Geometry check sheet. Reference: the model listing, model coordinates, mm. A direction names the side the tool comes from. Give positions to 0.01 mm unless a question says otherwise; leave off trailing zeros. Order: outer loops, then holes, each group sorted by start corner. A loop starts at its lowest first (then second) coordinate and runs counter-clockwise, first axis right, second up.
from build123d import *

# Parameters (mm, degrees)
F1_DEPTH = 25
F2_R     = 3
F3_DEPTH = 15


with BuildPart() as f1:
    # F0 (on Top) → F1 (new body)
    with BuildSketch(Plane.XY):
        with BuildLine():
            Line((5.183941, -22.5), (6.75, -22.5))
            ThreePointArc((6.75, -22.5), (7.28033, -22.28033), (7.5, -21.75))
            Line((7.5, -21.75), (7.5, 22.178048))
            ThreePointArc((7.5, 22.178048), (7.466599, 22.492831), (7.367882, 22.793595))
            Line((7.367882, 22.793595), (3, 32.5))
            Line((3, 32.5), (3, 77.5))
            Line((3, 77.5), (-3, 77.5))
            Line((-3, 77.5), (-3, 32.5))
            Line((-3, 32.5), (-7.367882, 22.793595))
            ThreePointArc((-7.367882, 22.793595), (-7.466599, 22.492831), (-7.5, 22.178048))
            Line((-7.5, 22.178048), (-7.5, -21.75))
            ThreePointArc((-7.5, -21.75), (-7.28033, -22.28033), (-6.75, -22.5))
            Line((-6.75, -22.5), (-5.316059, -22.5))
            ThreePointArc((-5.316059, -22.5), (-4.785729, -22.28033), (-4.566059, -21.75))
            Line((-4.566059, -21.75), (-4.566059, 22.03125))
            ThreePointArc((-4.566059, 22.03125), (-4.532658, 22.346033), (-4.433941, 22.646797))
            Line((-4.433941, 22.646797), (-0.683941, 30.980131))
            ThreePointArc((-0.683941, 30.980131), (0, 31.422357), (0.683941, 30.980131))
            Line((0.683941, 30.980131), (4.301823, 22.940392))
            ThreePointArc((4.301823, 22.940392), (4.40054, 22.639628), (4.433941, 22.324845))
            Line((4.433941, 22.324845), (4.433941, -21.75))
            ThreePointArc((4.433941, -21.75), (4.653611, -22.28033), (5.183941, -22.5))
        make_face()
    extrude(amount=F1_DEPTH)

    # F2 (on face) → F3 (cut)
    with BuildSketch(Plane.YZ.offset(7.5)):
        with BuildLine():
            Line((77.5, 25), (50.400115, 25))
            ThreePointArc((50.400115, 25), (51.768982, 24.874022), (53.091863, 24.500321))
            Line((53.091863, 24.500321), (73.81722, 16.531051))
            ThreePointArc((73.81722, 16.531051), (75.005426, 16.579196), (75.78519, 17.477038))
            ThreePointArc((75.78519, 17.477038), (76.5, 18), (77.21481, 17.477038))
            Line((77.21481, 17.477038), (77.5, 16.579144))
            Line((77.5, 16.579144), (77.5, 25))
        make_face()
        with BuildLine():
            Line((-21.75, 25), (-21.828302, 25))
            Line((-21.828302, 25), (-23.686077, 25))
            Line((-23.686077, 25), (-23.686077, 18))
            Line((-23.686077, 18), (-21.828302, 18))
            Line((-21.828302, 18), (41.671698, 18))
            ThreePointArc((41.671698, 18), (42.468668, 18.229237), (43.022045, 18.846881))
            ThreePointArc((43.022045, 18.846881), (43.089574, 19.175113), (43.171698, 19.5))
            ThreePointArc((43.171698, 19.5), (45.858639, 23.468668), (50.400115, 25))
            Line((50.400115, 25), (43.171698, 25))
            Line((43.171698, 25), (-21.75, 25))
        make_face()
        with BuildLine():
            ThreePointArc((43.022045, 18.846881), (43.133806, 19.164977), (43.171698, 19.5))
            ThreePointArc((43.171698, 19.5), (43.089574, 19.175113), (43.022045, 18.846881))
        make_face()
        with Locations((50.400115, 17.5)):
            Circle(F2_R)
        with Locations((-12.5, 10)):
            Circle(F2_R)
        with Locations((72.5, 11.531051)):
            Circle(F2_R)
    extrude(amount=-F3_DEPTH, mode=Mode.SUBTRACT)


solid = f1.part
Item 1: Sectioned sample at D-D (x = 2). Enter the section's corners in (y, z), and give its area (3 significant figures).
Reported:
outline: (28.06, 0) - (77.5, 0) - (77.5, 16.58) - (77.21, 17.48) arc R0.75 ccw to (75.79, 17.48) arc R1.5 cw to (73.82, 16.53) - (53.09, 24.5) arc R7.5 ccw to (50.4, 25) arc R7.5 ccw to (43.17, 19.5) arc R1.5 cw to (43.02, 18.85) arc R1.5 cw to (41.67, 18) - (28.06, 18) - close; hole circle Ø6 at (50.4, 17.5); hole circle Ø6 at (72.5, 11.53)
area: 942 mm2
Item 2: Sectioned sample at C-C (z = 10). Give the number of separate pieces and of enclosed holes in the cut face, and give its area (3 significant figures).
Reported:
separate pieces: 4
enclosed holes: 0
area: 533 mm2
Item 3: Scan lines: L1, parallel to X at y = 5.5, z = 8.75; L2, parallel to Z at x = -2.5, y = 41; L3, parallel to X at y = 45, z = 12. Record each from-to range of solid material in increasing order.
Reported:
L1: x = -7.5 to -4.57, 4.43 to 7.5
L2: z = 0 to 18
L3: x = -3 to 3
Item 4: Sectioned sample at A-A (y = -12.5). Enter the section's corners in (x, z).
Reported:
outline: (-7.5, 0) - (-4.57, 0) - (-4.57, 7) - (-7.5, 7) - close; (-7.5, 13) - (-4.57, 13) - (-4.57, 18) - (-7.5, 18) - close; (4.43, 0) - (7.5, 0) - (7.5, 7) - (4.43, 7) - close; (4.43, 13) - (7.5, 13) - (7.5, 18) - (4.43, 18) - close
Item 5: Set-up check for faces 1 (the flat face through (6, -22.5, 9)), 2 (the flat face through (2.468, 27.017, 8.874)), 3 (the flat face through (5, 9, 18)): record each of +Z, -Z, +X, -X, +Y, -Y from which the full face is reachable in a straight line by a thin tool's end or side.
Reported:
face 1: +Z, -Z, +X, -X, -Y
face 2: +Z, -Z, -Y
face 3: +Z, +X, -X, -Y
Item 6: Sectioned sample at B-B (y = 6). Enter the section's corners in (x, z).
Reported:
outline: (-7.5, 0) - (-4.57, 0) - (-4.57, 18) - (-7.5, 18) - close; (4.43, 0) - (7.5, 0) - (7.5, 18) - (4.43, 18) - close
Item 7: Gauge pin test, flat ends, axial feed: pin 1 (4 mm diameter, centred on x = -4, y = 61, fed in from -Z); pin 2 (3.5 mm diameter, centred on y = 50.4, z = 17.5, fed in from +X); pin 3 (3 mm diameter, centred on x = 0.5, z = 16, fed in from -Y); pin 4 (5 mm diameter, centred on x = -4.5, z = 19, fed in from +Y). Record the tip position at first contact, or that the pin passes through.
Reported:
pin 1: stops at z = 0
pin 2: passes through
pin 3: stops at y = 28.06
pin 4: stops at y = 77.37
Item 8: Draft check along Z on faces 4 (the flat face through (-3, 55, 10)), 5 (the cylindrical face through (0.042, 51.75, 24.878)), 6 (the cylindrical face through (6, -14.9, 8.2)). Enter one of: released by +Z, released by -Z, zero draft, split by the parting line, or undercut.
Reported:
face 4: zero draft
face 5: released by +Z
face 6: undercut
